Autodesk Inventor part; units mm, degrees
ref_plane "YZ Plane" through (0, 0, 0) normal (1, 0, 0) x (0, 1, 0)
ref_plane "XZ Plane" through (0, 0, 0) normal (0, 1, 0) x (-1, 0, 0)
ref_plane "XY Plane" through (0, 0, 0) normal (0, 0, 1) x (1, 0, 0)
sketch "Szkic1" plane through (0, 0, 0) normal (0, 0, 1) x (1, 0, 0)
  circle A0 centre (0, 0) radius 20
  circle A1 centre (10.6, 10.6) radius 2.15
  circle A2 centre (-10.6, 10.6) radius 2.15
  circle A3 centre (-10.6, -10.6) radius 2.15
  circle A4 centre (10.6, -10.6) radius 2.15
  arc A5 (1.8342, -1.954) -> (-1.8342, -1.954) centre (0, 0) ccw
  line L0 (0, -1.954) -> (1.8342, -1.954)
  line L1 (0, -1.954) -> (-1.8342, -1.954)
  dimension "d0" = 40
  dimension "d3" = 4.3
  dimension "d6" = 360
  dimension "d8" = 5.36
extrude "Wyciągnięcie proste1" add sketch "Szkic1" along normal blind 4
sketch "Szkic2" plane through (0, 0, 4) normal (0, 0, 1) x (1, 0, 0)
  arc A0 (5.9908, -3) -> (-6.0091, -2.9632) centre (0, 0) ccw
  circle A1 centre (0, 0) radius 20
  line L0 (0, -10) -> (6, -10)
  line L1 (6, -10) -> (5.9908, -3)
  line L2 (5.9908, -3) -> (-6.0091, -2.9632)
  line L3 (-6.0091, -2.9632) -> (-6.0091, -9.9632)
  line L4 (-6.0091, -9.9632) -> (0, -10)
  line L5 (-0.0091, -3.6816) -> (2.8909, -3.6816)
  line L6 (2.8909, -3.6816) -> (2.8909, -6.4816)
  line L7 (2.8909, -6.4816) -> (-2.9091, -6.4816)
  line L8 (-2.9091, -6.4816) -> (-2.9091, -3.6816)
  line L9 (-2.9091, -3.6816) -> (-0.0091, -3.6816)
  dimension "d12" = 13.4
  dimension "d19" = 6
  dimension "d20" = 7
  dimension "d21" = 12
  dimension "d24" = 7
  dimension "d26" = 2.9
  dimension "d27" = 2.8
  dimension "d28" = 5.8
extrude "Wyciągnięcie proste2" add sketch "Szkic2" along normal blind 8 contours L1 L0 L4 L3 L2
sketch "Szkic3" plane through (0, 0, 4) normal (0, 0, 1) x (1, 0, 0)
  circle A0 centre (0, 0) radius 6.7
  line L0 (-6.0091, -9.9632) -> (-6.0091, -2.9632)
  line L1 (6, -10) -> (5.9908, -3)
  line L2 (-6.0091, -2.9632) -> (5.9908, -3)
  dimension "d31" = 13.4
sketch "Szkic4" plane through (0, 0, 4) normal (0, 0, 1) x (1, 0, 0)
  arc A0 (1.8342, -1.954) -> (-1.8342, -1.954) centre (0, 0) ccw
  line L0 (-1.8342, -1.954) -> (1.8342, -1.954)
  arc A1 (1.8342, -1.954) -> (-1.8342, -1.954) centre (0, 0) ccw
sketch "Szkic5" plane through (0, 0, 4) normal (0, 0, 1) x (1, 0, 0)
  point P0 (0, 0)
extrude "Wyciągnięcie proste3" add sketch "Szkic3" along normal blind 8 contours A0 L2 picked at (-1.2468, -0.1308)
extrude "Wyciągnięcie proste4" cut sketch "Szkic4" along normal blind 8
sketch "Szkic6" plane through (0, -10, 4) normal (-0.0061262, -0.9999812, 0) x (0.9999812, -0.0061262, 0)
  circle A0 centre (0, 4) radius 1.6
  point P0 (-0.0613, -4)
  point P1 (0, 0)
  dimension "d37" = 3.2
extrude "Wyciągnięcie proste5" cut sketch "Szkic6" against normal blind 8
sketch "Szkic7" plane through (0.049, -2.0002, 8) normal (-0.0061262, -0.9999812, 0) x (0.9999812, -0.0061262, 0)
  point P0 (-0.0613, -8)
sketch "Szkic8" plane through (0.049, -2.0002, 8) normal (-0.0061262, -0.9999812, 0) x (0.9999812, -0.0061262, 0)
  circle A0 centre (0, 0) radius 1.6
  point P0 (-0.0613, -8)
  dimension "d40" = 3.2
extrude "Wyciągnięcie proste6" cut sketch "Szkic8" against normal blind 2
fillet "Zaokrąglenie1" radius 4 1 edges at (-6.0091, -9.9632, 8)
fillet "Zaokrąglenie2" radius 4 1 edges at (6, -10, 8)
sketch "Szkic9" plane through (0, -10, 8) normal (-0.0061262, -0.9999812, 0) x (0.9999812, -0.0061262, 0)
  point P0 (-0.0613, -8)
properties part number "sprzeglo"
For this review, take the finished solid that the model builds, in its own axes (mm). A direction names the side the tool comes from. Give positions to 0.01 mm unless a question says otherwise; leave off trailing zeros. Write each loop counter-clockwise with the first axis right and the second up, starting at its lowest first coordinate (ties: lowest second). Pieces come first, ordered by that corner, then holes.
Item 1: Take a section at A-A (y = 0). Give the boundary of the cut face in (x, z).
Item 2: Take a section at B-B (z = 3.25). Give the boundary of the cut face in (x, y), and give its area (3 significant figures).
Item 3: Machinability: for faces 5 (the face through (0, -5, 4)), 6 (the face through (-6.009, -4, 8)), 7 (the face through (0, -1.954, 6)), which of the approach directions +Z, -Z, +X, -X, +Y, -Y give a long, thin tool a straight path to every point of the face, cutting with its end or side? Answer none if there is none.
Item 4: Insertion check: P1, Ø4, axis at x = -10.6, y = 10.6, coming from the -Z side; P2, Ø4, axis at x = -11, z = 1.5, coming from the +Y side; P3, Ø1.1, axis at x = -0.5, z = 5, coming from the +Y side; P4, Ø1.5, axis at x = 13, y = -9, coming from the +Z side. Each pin has a flat end and moves straight along its axis. Give the tip position at first contact, or say it passes through.
Item 5: Take a section at C-C (x = 10.6). Give the boundary of the cut face in (y, z).
Item 6: The part is to be moulded in two halves that separate along X. For faces 1 (the face through (4, 0, 0)), 2 (the face through (-0.17, 6.698, 7.944)), 3 (the face through (-4.877, -8.776, 8.056)), 4 (the face through (-11.07, -8.5, 1.97)), say which applies: +X half, -X half, draft (parallel to the pull), parting line (faces both ways), or undercut.
Item 7: Wall thickness on probe 1 along X at (y, z) = (0, 9.25); probe 2 along X at (y, z) = (-10.5, 3.5); probe 3 along Y at (x, z) = (-9, 1): over which ranges is each line inside the solid? List them lowest first.
Established:
1. outline: (-20, 0) - (-2.68, 0) - (-2.68, 12) - (-6.7, 12) - (-6.7, 4) - (-20, 4) - close; (2.68, 0) - (20, 0) - (20, 4) - (6.7, 4) - (6.7, 12) - (2.68, 12) - close
2. outline: circle Ø40 at (0, 0); hole circle Ø4.3 at (-10.6, -10.6); hole circle Ø4.3 at (-10.6, 10.6); hole (-1.83, -1.95) - (1.83, -1.95) arc R2.68 ccw (long way) to start; hole circle Ø4.3 at (10.6, -10.6); hole circle Ø4.3 at (10.6, 10.6)
2. area: 1,180 mm2
3. face 5: +Z
3. face 6: +Z, -X, -Y
3. face 7: +Z, -Z
4. P1: passes through
4. P2: stops at y = 17.86
4. P3: stops at y = 6.7
4. P4: stops at z = 4
5. outline: (-16.96, 0) - (-12.75, 0) - (-12.75, 4) - (-16.96, 4) - close; (-8.45, 0) - (8.45, 0) - (8.45, 4) - (-8.45, 4) - close; (12.75, 0) - (16.96, 0) - (16.96, 4) - (12.75, 4) - close
6. face 1: draft
6. face 2: parting line
6. face 3: -X half
6. face 4: undercut
7. probe 1: x = -6.7 to -2.68, 2.68 to 6.7
7. probe 2: x = -17.02 to -12.75, -8.45 to 8.45, 12.75 to 17.02
7. probe 3: y = -17.86 to -12.04, -9.16 to 9.16, 12.04 to 17.86
